```python
from build123d import *

# Parameters (mm, degrees)
SKETCH_1_R                       = 2.1
SM_BASE_FLANGE_1_DEPTH           = 2
SM_EDGE_FLANGE_1_STRIP_W         = 12
SM_EDGE_FLANGE_1_STRIP_H         = 2
SM_EDGE_FLANGE_1_STRIP_CUT_DEPTH = 55
SM_EDGE_FLANGE_1_DEPTH           = 55
SM_EDGE_FLANGE_2_STRIP_W         = 12
SM_EDGE_FLANGE_2_STRIP_H         = 2
SM_EDGE_FLANGE_2_STRIP_CUT_DEPTH = 55
SM_EDGE_FLANGE_2_DEPTH           = 55
SM_EDGE_FLANGE_2_PROFILE_R       = 2.5
SM_EDGE_FLANGE_2_FLAT_DEPTH      = 2
SKETCH_12_R                      = 3
EXTRUDE_1_DEPTH                  = 2
HOLE_WIZARD_M4_1_D               = 3.3
HOLE_WIZARD_M4_1_DEPTH           = 6
HOLE_WIZARD_M4_1_TIP             = 0.991420021


# Sheet-metal steps are written as plain solids
with BuildPart() as part:
    # Sketch 1 → 基体-法兰1 (new body)
    with BuildSketch(Plane.XY):
        with BuildLine():
            Line((-27.5, 20), (27.5, 20))
            Line((27.5, 20), (27.5, -10))
            ThreePointArc((27.5, -10), (24.571067812, -17.071067812), (17.5, -20))
            Line((17.5, -20), (-17.5, -20))
            ThreePointArc((-17.5, -20), (-24.571067812, -17.071067812), (-27.5, -10))
            Line((-27.5, -10), (-27.5, 20))
        make_face()
        with Locations((-17.5, 10)):
            Circle(SKETCH_1_R, mode=Mode.SUBTRACT)
        with Locations(Location((17.5, 10, 0), (0, 0, 180))):
            Circle(SKETCH_1_R, mode=Mode.SUBTRACT)
        with Locations((17.5, -10)):
            Circle(SKETCH_1_R, mode=Mode.SUBTRACT)
        with Locations(Location((-17.5, -10, 0), (0, 0, 180))):
            Circle(SKETCH_1_R, mode=Mode.SUBTRACT)
        with Locations((-17.5, 0)):
            Circle(SKETCH_1_R, mode=Mode.SUBTRACT)
        with Locations((17.5, 0)):
            Circle(SKETCH_1_R, mode=Mode.SUBTRACT)
    extrude(amount=-SM_BASE_FLANGE_1_DEPTH)

    # 边线-法兰1 strip (across the edge) → 边线-法兰1 strip cut (cut)
    with BuildSketch(Plane(origin=(27.5, 20, 0), x_dir=(0, -1, 0), z_dir=(-1, 0, 0))):
        with Locations((-2, -1)):
            Rectangle(SM_EDGE_FLANGE_1_STRIP_W, SM_EDGE_FLANGE_1_STRIP_H)
    extrude(amount=SM_EDGE_FLANGE_1_STRIP_CUT_DEPTH, mode=Mode.SUBTRACT)

    # 边线-法兰1 section (across the edge) → 边线-法兰1 (add)
    with BuildSketch(Plane(origin=(27.5, 20, 0), x_dir=(0, -1, 0), z_dir=(-1, 0, 0))):
        with BuildLine():
            Line((0, 2), (0, 63.8))
            Line((0, 63.8), (2, 63.8))
            Line((2, 63.8), (2, 2))
            ThreePointArc((2, 2), (2.585786438, 0.585786438), (4, 0))
            Line((4, 0), (4, -2))
            ThreePointArc((4, -2), (1.171572875, -0.828427125), (0, 2))
        make_face()
    extrude(amount=SM_EDGE_FLANGE_1_DEPTH)

    # 边线-法兰2 strip (across the edge) → 边线-法兰2 strip cut (cut)
    with BuildSketch(Plane(origin=(27.5, 18, 63.8), x_dir=(0, 0, -1), z_dir=(-1, 0, 0))):
        with Locations((-2, -1)):
            Rectangle(SM_EDGE_FLANGE_2_STRIP_W, SM_EDGE_FLANGE_2_STRIP_H)
    extrude(amount=SM_EDGE_FLANGE_2_STRIP_CUT_DEPTH, mode=Mode.SUBTRACT)

    # 边线-法兰2 bend section (across the edge) → 边线-法兰2 (add)
    with BuildSketch(Plane(origin=(27.5, 18, 63.8), x_dir=(0, 0, -1), z_dir=(-1, 0, 0))):
        with BuildLine():
            Line((0, 2), (2, 2))
            ThreePointArc((2, 2), (2.585786438, 0.585786438), (4, 0))
            Line((4, 0), (4, -2))
            ThreePointArc((4, -2), (1.171572875, -0.828427125), (0, 2))
        make_face()
    extrude(amount=SM_EDGE_FLANGE_2_DEPTH)

    # 边线-法兰2 profile (on flange) → 边线-法兰2 flat (add)
    with BuildSketch(Plane(origin=(0, 18, 63.8), x_dir=(-1, 0, 0), z_dir=(0, 0, 1))):
        with BuildLine():
            Line((-27.5, 2), (27.5, 2))
            Line((27.5, 2), (27.5, 25.8))
            ThreePointArc((27.5, 25.8), (24.571067812, 32.871067812), (17.5, 35.8))
            Line((17.5, 35.8), (-17.5, 35.8))
            ThreePointArc((-17.5, 35.8), (-24.571067812, 32.871067812), (-27.5, 25.8))
            Line((-27.5, 25.8), (-27.5, 2))
        make_face()
        with Locations((17.5, 8)):
            Circle(SM_EDGE_FLANGE_2_PROFILE_R, mode=Mode.SUBTRACT)
        with Locations((17.5, 18)):
            Circle(SM_EDGE_FLANGE_2_PROFILE_R, mode=Mode.SUBTRACT)
        with Locations((-17.5, 8)):
            Circle(SM_EDGE_FLANGE_2_PROFILE_R, mode=Mode.SUBTRACT)
        with Locations((-17.5, 18)):
            Circle(SM_EDGE_FLANGE_2_PROFILE_R, mode=Mode.SUBTRACT)
        with Locations((17.5, 28)):
            Circle(SM_EDGE_FLANGE_2_PROFILE_R, mode=Mode.SUBTRACT)
        with Locations((-17.5, 28)):
            Circle(SM_EDGE_FLANGE_2_PROFILE_R, mode=Mode.SUBTRACT)
    extrude(amount=-SM_EDGE_FLANGE_2_FLAT_DEPTH)

    # 草图12 → 凸台-拉伸1 (add)
    with BuildSketch(Plane(origin=(0, 0, 61.8), x_dir=(-1, 0, 0), z_dir=(0, 0, -1))):
        with Locations(Location((0, 0, 0), (0, 0, 270))):
            Circle(SKETCH_12_R)
    extrude(amount=EXTRUDE_1_DEPTH)

    # M4 螺纹孔1
    with Locations(Plane.XY.offset(63.8)):
        with Locations((0, 0)):
            Hole(HOLE_WIZARD_M4_1_D / 2, depth=HOLE_WIZARD_M4_1_DEPTH)
            with Locations((0, 0, -(HOLE_WIZARD_M4_1_DEPTH + HOLE_WIZARD_M4_1_TIP / 2))):  # 118° drill point
                Cone(0, HOLE_WIZARD_M4_1_D / 2, HOLE_WIZARD_M4_1_TIP, mode=Mode.SUBTRACT)


solid = part.part
```
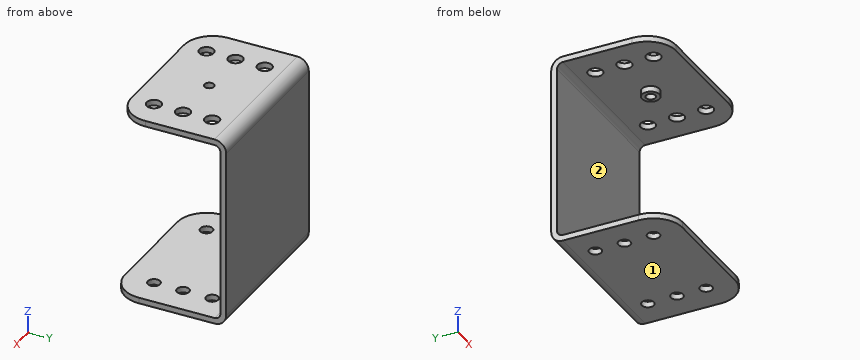
The model under review builds one solid part; all positions refer to its coordinate system, in mm. Face numbers are marked on the shaded views. A direction names the side the tool comes from. Round coordinates to 2 decimals unless told otherwise and drop trailing zeros. Order: outer loops, then holes, each group sorted by start corner. A loop starts at its lowest first (then second) coordinate and runs counter-clockwise, first axis right, second up.
Item 1: Add section A-A, the plane y = 10. State the section outline as (x, z) points.
Working result:
outline: (-27.5, -2) - (-19.6, -2) - (-19.6, 0) - (-27.5, 0) - close; (-27.5, 61.8) - (-20, 61.8) - (-20, 63.8) - (-27.5, 63.8) - close; (-15.4, -2) - (15.4, -2) - (15.4, 0) - (-15.4, 0) - close; (-15, 61.8) - (15, 61.8) - (15, 63.8) - (-15, 63.8) - close; (19.6, -2) - (27.5, -2) - (27.5, 0) - (19.6, 0) - close; (20, 61.8) - (27.5, 61.8) - (27.5, 63.8) - (20, 63.8) - close
Item 2: Add section C-C, the plane x = -12.5. State the section outline as (y, z) points, and give its area (3 significant figures).
Working result:
outline: (-20, -2) - (16, -2) arc R4 ccw to (20, 2) - (20, 59.8) arc R4 ccw to (16, 63.8) - (-17.8, 63.8) - (-17.8, 61.8) - (16, 61.8) arc R2 cw to (18, 59.8) - (18, 2) arc R2 cw to (16, 0) - (-20, 0) - close
area: 274 mm2
Item 3: Add section B-B, the plane y = 0. Count the separate pieces of the cut face and the enclosed holes in it, and give its area (3 significant figures).
Working result:
separate pieces: 7
enclosed holes: 0
area: 182 mm2
Item 4: For pin 1 (3.5 mm diameter, centred on x = 17.5, y = 0, fed in from -Z); pin 2 (16.5 mm diameter, centred on x = 12, z = 30, fed in from -Y); pin 3 (0.6 mm diameter, centred on x = 7, z = 63, fed in from -Y), all flat-tipped, find the tip position at first contact; note any pin that passes through.
Working result:
pin 1: passes through
pin 2: stops at y = 18
pin 3: stops at y = -17.8
Item 5: Add section D-D, the plane y = -17. State the section outline as (x, z) points, and give its area (3 significant figures).
Working result:
outline: (-24.64, -2) - (24.64, -2) - (24.64, 0) - (-24.64, 0) - close; (-21.42, 61.8) - (21.42, 61.8) - (21.42, 63.8) - (-21.42, 63.8) - close
area: 184 mm2
Item 6: To check wall thickness, follow probe 1 along Z at (x, y) = (10, 3); probe 2 along Y at (x, z) = (-17.5, 63.1); probe 3 along X at (y, z) = (-10, 63.1) (3 decimals). State the ranges of each line that lie inside material, in increasing order.
Working result:
probe 1: z = -2 to 0, 61.8 to 63.8
probe 2: y = -17.8 to -12.5, -7.5 to -2.5, 2.5 to 7.5, 12.5 to 18.26
probe 3: x = -27.255 to -20, -15 to 15, 20 to 27.255
Item 7: Machinability: for the marked faces 1 and 2, which of the approach directions +Z, -Z, +X, -X, +Y, -Y give a long, thin tool a straight path to every point of the face, cutting with its end or side? Answer none if there is none.
Working result:
face 1: -Z, +X, -X, +Y, -Y
face 2: +X, -X, -Y
